from build123d import *

# Parameters (mm, degrees)
F1_DEPTH       = 5.08
F3_D           = 4.445
F3_CSINK_D     = 7.62
F3_CSINK_ANGLE = 90
F4_T1_DEPTH    = 101.4234647155
F4_T3_DEPTH    = 19.05
F4_T5_DEPTH    = 19.05
F4_T7_DEPTH    = 18.1679810636
F4_T10_ANGLE   = 90
F4_T12_ANGLE   = 90
F5_W           = 25.4
F5_H           = 6.35
F6_DEPTH       = 1.27


# Not quite as in the source:
# - a fillet or chamfer that OpenCascade refuses, or shapes differently, is made with other operations: its cross-section is extruded or revolved along the edge and cut away or added


with BuildPart() as f1:
    # F0 (on Front) → F1 (new body, symmetric)
    with BuildSketch(Plane.XZ):
        with BuildLine():
            Line((50.7117323577, 0), (0, 0))
            Line((0, 0), (-50.7117323577, 0))
            ThreePointArc((-50.7117323577, 0), (-57.2033226337, 2.6889047337), (-59.8922273673, 9.1804950096))
            Line((-59.8922273673, 9.1804950096), (-59.8922273673, 20.9984760731))
            Line((-59.8922273673, 20.9984760731), (-66.2422273673, 20.9984760731))
            Line((-66.2422273673, 20.9984760731), (-66.2422273673, 9.1804950096))
            ThreePointArc((-66.2422273673, 9.1804950096), (-61.6934506942, -1.8012233269), (-50.7117323577, -6.35))
            Line((-50.7117323577, -6.35), (0, -6.35))
            Line((0, -6.35), (50.7117323577, -6.35))
            ThreePointArc((50.7117323577, -6.35), (61.6934506942, -1.8012233269), (66.2422273673, 9.1804950096))
            Line((66.2422273673, 9.1804950096), (66.2422273673, 20.9984760731))
            Line((66.2422273673, 20.9984760731), (59.8922273673, 20.9984760731))
            Line((59.8922273673, 20.9984760731), (59.8922273673, 9.1804950096))
            ThreePointArc((59.8922273673, 9.1804950096), (57.2033226337, 2.6889047337), (50.7117323577, 0))
        make_face()
    extrude(amount=F1_DEPTH, both=True)

    # F3 (through all)
    with Locations(Plane(origin=(0, 0, -6.35), x_dir=(1, 0, 0), z_dir=(0, 0, -1))):
        with Locations((-46.4819967747, 0), (46.443849802, 0)):
            CounterSinkHole(F3_D / 2, F3_CSINK_D / 2, counter_sink_angle=F3_CSINK_ANGLE)

    # F4: fillet of radius 2.54 on 7 edges, made by hand

    # F4_s2 → F4_t1 (cut)
    with BuildSketch(Plane.YZ.offset(-50.7117323577)):
        with BuildLine():
            ThreePointArc((5.08, -3.81), (4.3360512242, -5.6060512242), (2.54, -6.35))
            Line((2.54, -6.35), (5.08, -6.35))
            Line((5.08, -6.35), (5.08, -3.81))
        make_face()
    extrude(amount=F4_T1_DEPTH, mode=Mode.SUBTRACT)

    # F4_s4 → F4_t3 (cut)
    with BuildSketch(Plane.YZ.offset(53.5422273673)):
        with BuildLine():
            ThreePointArc((5.08, 18.4584760731), (4.3360512242, 20.2545272974), (2.54, 20.9984760731))
            Line((2.54, 20.9984760731), (5.08, 20.9984760731))
            Line((5.08, 20.9984760731), (5.08, 18.4584760731))
        make_face()
    extrude(amount=F4_T3_DEPTH, mode=Mode.SUBTRACT)

    # F4_s6 → F4_t5 (cut)
    with BuildSketch(Plane.YZ.offset(-72.5922273673)):
        with BuildLine():
            ThreePointArc((5.08, 18.4584760731), (4.3360512242, 20.2545272974), (2.54, 20.9984760731))
            Line((2.54, 20.9984760731), (5.08, 20.9984760731))
            Line((5.08, 20.9984760731), (5.08, 18.4584760731))
        make_face()
    extrude(amount=F4_T5_DEPTH, mode=Mode.SUBTRACT)

    # F4_s8 → F4_t7 (cut)
    with BuildSketch(Plane.XY.offset(9.1804950096)):
        with BuildLine():
            ThreePointArc((63.7022273673, 5.08), (65.4982785915, 4.3360512242), (66.2422273673, 2.54))
            Line((66.2422273673, 2.54), (66.2422273673, 5.08))
            Line((66.2422273673, 5.08), (63.7022273673, 5.08))
        make_face()
        with BuildLine():
            ThreePointArc((-63.7022273673, 5.08), (-65.4982785915, 4.3360512242), (-66.2422273673, 2.54))
            Line((-66.2422273673, 2.54), (-66.2422273673, 5.08))
            Line((-66.2422273673, 5.08), (-63.7022273673, 5.08))
        make_face()
    extrude(amount=F4_T7_DEPTH, mode=Mode.SUBTRACT)

    # F4_s9 → F4_t10 (revolve, cut)
    with BuildSketch(Plane.YZ.offset(50.7117323577)):
        with BuildLine():
            ThreePointArc((2.54, -6.35), (4.3360512242, -5.6060512242), (5.08, -3.81))
            Line((5.08, -3.81), (5.08, -6.35))
            Line((5.08, -6.35), (2.54, -6.35))
        make_face()
    revolve(axis=Axis((50.7117323577, 5.08, 9.1804950096), (0, -1, 0)), revolution_arc=F4_T10_ANGLE, mode=Mode.SUBTRACT)

    # F4_s11 → F4_t12 (revolve, cut)
    with BuildSketch(Plane.XY.offset(9.1804950096)):
        with BuildLine():
            ThreePointArc((-63.7022273673, 5.08), (-65.4982785915, 4.3360512242), (-66.2422273673, 2.54))
            Line((-66.2422273673, 2.54), (-66.2422273673, 5.08))
            Line((-66.2422273673, 5.08), (-63.7022273673, 5.08))
        make_face()
    revolve(axis=Axis((-50.7117323577, 5.08, 9.1804950096), (0, -1, 0)), revolution_arc=F4_T12_ANGLE, mode=Mode.SUBTRACT)

    # F5 (on face) → F6 (join)
    with BuildSketch(Plane(origin=(0, 0, -6.35), x_dir=(1, 0, 0), z_dir=(0, 0, -1))):
        Rectangle(F5_W, F5_H)
    extrude(amount=F6_DEPTH)


solid = f1.part
Can you work these out from the model? Positions are in its coordinate system, mm. A direction names the side the tool comes from. Round coordinates to 2 decimals unless told otherwise and drop trailing zeros. Order: outer loops, then holes, each group sorted by start corner. A loop starts at its lowest first (then second) coordinate and runs counter-clockwise, first axis right, second up. Notation, with made-up numbers: M 70.25,84 L 128.25,84 A6 cw 128.25,89 Z; hole C -34.5,22.25 d10. An arc over 180 degrees is marked long. Use a Markdown table: item, result.
1) On a 3-axis mill with a long thin cutter (end or side, diameter ignored), from which of +Z, -Z, +X, -X, +Y, -Y can I reach the whole of each face in a straight line? I mean faces 1 (the face through (1, 0, 0)), 2 (the face through (44.39, 0.85, -2.35)). Say none if no direction works.
Geometry says:
| item | result |
|---|---|
| face 1 | +Z, +Y, -Y |
| face 2 | +Z, -Z |
2) If I drill on line 1 along X through (y, z) = (-1.5, 14.5); line 2 along Z through (x, y) = (-17.5, -4.5); line 3 along X through (y, z) = (-4, 2.75), over which ranges is the centre line in solid material (lowest first)?
Geometry says:
| item | result |
|---|---|
| line 1 | x = -66.24 to -59.89, 59.89 to 66.24 |
| line 2 | z = -6.35 to 0 |
| line 3 | x = -64.85 to -57.26, 57.26 to 64.85 |
3) If we mould it in two halves opening along X, with no side actions, what happens to faces 3 (the face through (-66.242, -1, 15)), 4 (the face through (-63, -1, 20.998)), 5 (the face through (-48.535, 0.851, -2.348))? For each: +X half, -X half, draft (parallel to the pull), parting line (faces both ways), or undercut.
Geometry says:
| item | result |
|---|---|
| face 3 | -X half |
| face 4 | draft |
| face 5 | undercut |
4) I'm going to push flat-ended pins straight in: P1, Ø4, axis at x = -15.5, y = -1, coming from the -Z side; P2, Ø6, axis at x = -27, y = 2.5, coming from the +Z side; P3, Ø1, axis at y = -0.5, z = -7, coming from the +X side; P4, Ø4, axis at x = 46.44, y = 0, coming from the -Z side. Where does each tip first touch, or does it pass through?
Geometry says:
| item | result |
|---|---|
| P1 | stops at z = -6.35 |
| P2 | stops at z = 0 |
| P3 | stops at x = 12.7 |
| P4 | passes through |
5) Imagine slicing it at C-C (x = -23.5). List the corners of the cut face in (y, z) for me.
Geometry says:
| item | result |
|---|---|
| outline | M -5.08,-6.35 L 2.54,-6.35 A2.54 ccw 5.08,-3.81 L 5.08,0 L -5.08,0 Z |
6) Imagine slicing it at A-A (y = 0). List the corners of the cut face in (x, z) for me, then the cut area to 3 significant figures.
Geometry says:
| item | result |
|---|---|
| outline | M -66.24,9.18 A15.53 ccw -50.71,-6.35 L -50.29,-6.35 L -48.7,-4.76 L -48.7,0 L -50.71,0 A9.18 cw -59.89,9.18 L -59.89,21 L -66.24,21 Z; M -44.26,-4.76 L -42.67,-6.35 L -12.7,-6.35 L -12.7,-7.62 L 12.7,-7.62 L 12.7,-6.35 L 42.63,-6.35 L 44.22,-4.76 L 44.22,0 L -44.26,0 Z; M 48.67,-4.76 L 50.25,-6.35 L 50.71,-6.35 A15.53 ccw 66.24,9.18 L 66.24,21 L 59.89,21 L 59.89,9.18 A9.18 cw 50.71,0 L 48.67,0 Z |
| area | 1,010 mm² |
7) Imagine slicing it at B-B (x = 0). List the corners of the cut face in (y, z) for me (3 decimals).
Geometry says:
| item | result |
|---|---|
| outline | M -5.08,-6.35 L -3.175,-6.35 L -3.175,-7.62 L 3.175,-7.62 L 3.175,-6.35 L 2.54,-6.35 A2.54 ccw 5.08,-3.81 L 5.08,0 L -5.08,0 Z |
